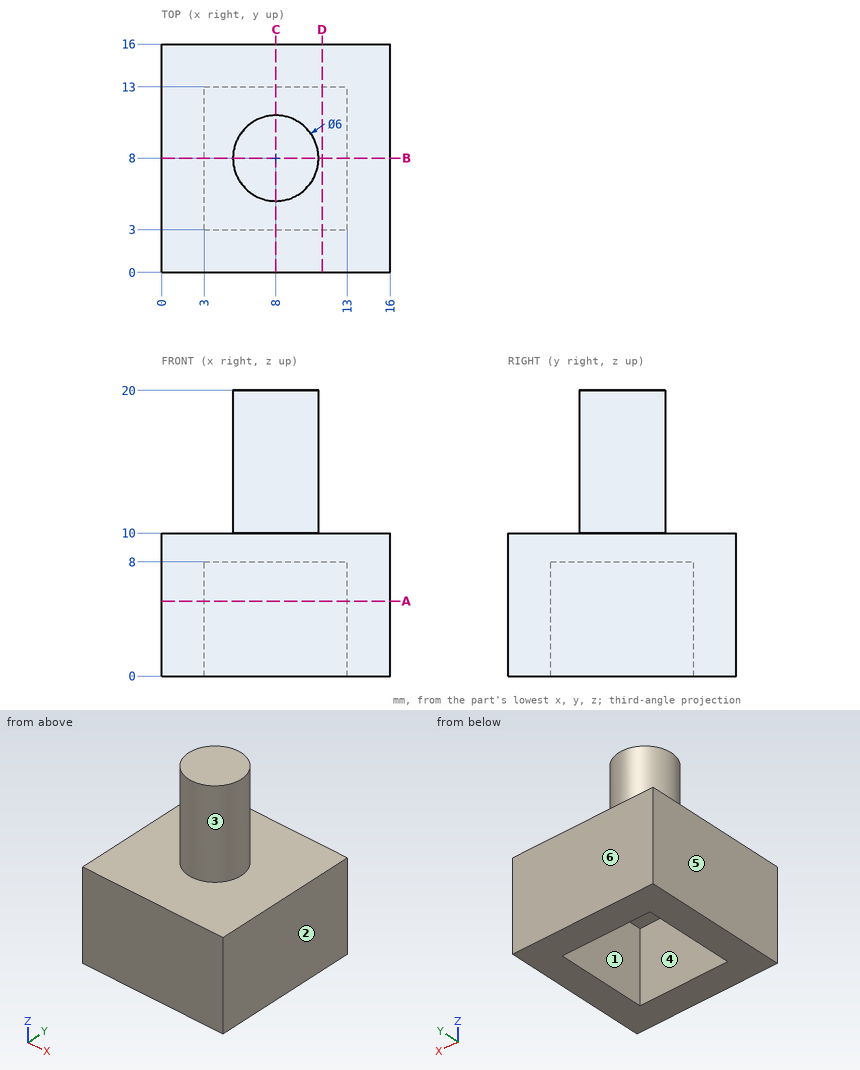
Geometry check sheet. Reference: drawing and pictorial views, mm from the part's lowest x, y, z. A direction names the side the tool comes from. Coordinates: 2 decimals unless noted, no trailing zeros. Write each loop counter-clockwise with the first axis right and the second up, starting at its lowest first coordinate (ties: lowest second). Pieces come first, ordered by that corner, then holes. Notation, with made-up numbers: M 11.25,39.5 L 33.25,39.5 A20 cw 33.25,76.5 Z; hole C 53.5,89 d1. An arc over 180 degrees is marked long. Use one line per item in the form item = value.
Item 1: Sectioned sample at A-A, the plane z = 5.25. Record the cut outline in (x, y), and give its area (3 significant figures).
Answer below:
outline = M 0,0 L 16,0 L 16,16 L 0,16 Z; hole M 3,3 L 13,3 L 13,13 L 3,13 Z
area = 156 mm^2
Item 2: Release check for a two-part mould opening along X. For the marked faces 4, 5 and 6 record: pulls with the +X half, pulls with the -X half, needs draft (parallel to the pull), parting line crosses it, or undercut.
Answer below:
face_4 = undercut
face_5 = pulls with the -X half
face_6 = needs draft
Item 3: Set-up check for the marked faces 1, 2 and 3: record each of +Z, -Z, +X, -X, +Y, -Y from which the full face is reachable in a straight line by a thin tool's end or side.
Answer below:
face_1 = -Z
face_2 = +Z, -Z, +X, +Y, -Y
face_3 = +Z
Item 4: Material ranges on L1, parallel to X at y = 12, z = 6; L2, parallel to Z at x = 11.5, y = 11.25, recorded low to high. Write a range as from..to.
Answer below:
L1 = 0..3, 13..16
L2 = 8..10
Item 5: Gauge pin test, flat ends, axial feed: pin 1 Ø8 at (y, z) = (11.5, 14.5) entering from -X; pin 2 Ø6.5 at (x, z) = (9, 4.5) entering from -Y. Record the tip position at first contact, or that the pin passes through.
Answer below:
pin_1 = 5
pin_2 = 0
Item 6: Sectioned sample at D-D, the plane x = 11.25. Record the cut outline in (y, z), and give its area (3 significant figures).
Answer below:
outline = M 0,0 L 3,0 L 3,8 L 13,8 L 13,0 L 16,0 L 16,10 L 0,10 Z
area = 80.0 mm^2
Item 7: Sectioned sample at B-B, the plane y = 8. Record the cut outline in (x, z).
Answer below:
outline = M 0,0 L 3,0 L 3,8 L 13,8 L 13,0 L 16,0 L 16,10 L 11,10 L 11,20 L 5,20 L 5,10 L 0,10 Z
